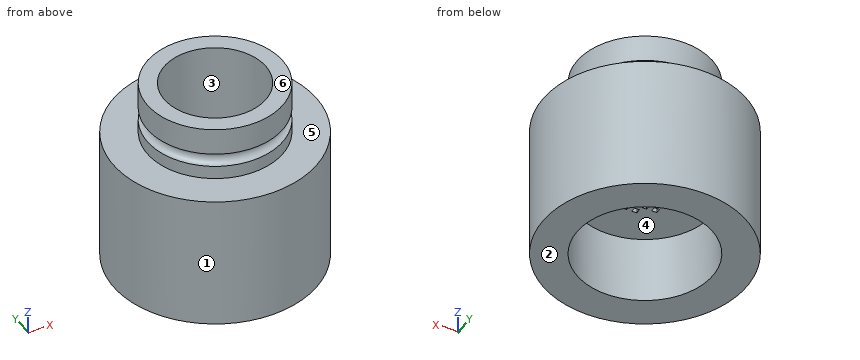
from build123d import *

# Parameters (mm, degrees)
SKETCH1_R                  = 15
BOSS_EXTRUDE1_DEPTH        = 10
SKETCH2_R                  = 10
CUT_EXTRUDE1_DEPTH         = 20
SKETCH3_R                  = 15
BOSS_EXTRUDE2_DEPTH        = 10
SKETCH5_R                  = 10
CUT_EXTRUDE3_DEPTH         = 8
SKETCH8_W                  = 0.75
SKETCH8_H                  = 0.75
CUT_EXTRUDE5_DEPTH         = 2
FILL_START                 = -1.125
FILL_PATTERN2_OUTLINE_W    = 0.75
FILL_PATTERN2_OUTLINE_H    = 2
FILL_PATTERN2_DEPTH        = 0.75
FILL_START_2               = 0.375
FILL_PATTERN2_2_OUTLINE_W  = 0.75
FILL_PATTERN2_2_OUTLINE_H  = 2
FILL_PATTERN2_2_DEPTH      = 0.75
FILL_START_3               = -3.375
FILL_PATTERN2_3_OUTLINE_W  = 0.75
FILL_PATTERN2_3_OUTLINE_H  = 2
FILL_PATTERN2_3_DEPTH      = 0.75
FILL_START_4               = -1.875
FILL_PATTERN2_4_OUTLINE_W  = 0.75
FILL_PATTERN2_4_OUTLINE_H  = 2
FILL_PATTERN2_4_DEPTH      = 0.75
FILL_START_5               = 1.125
FILL_PATTERN2_5_OUTLINE_W  = 0.75
FILL_PATTERN2_5_OUTLINE_H  = 2
FILL_PATTERN2_5_DEPTH      = 0.75
FILL_START_6               = 2.625
FILL_PATTERN2_6_OUTLINE_W  = 0.75
FILL_PATTERN2_6_OUTLINE_H  = 2
FILL_PATTERN2_6_DEPTH      = 0.75
FILL_START_7               = -4.125
FILL_PATTERN2_7_OUTLINE_W  = 0.75
FILL_PATTERN2_7_OUTLINE_H  = 2
FILL_PATTERN2_7_DEPTH      = 0.75
FILL_START_8               = -2.625
FILL_PATTERN2_8_OUTLINE_W  = 0.75
FILL_PATTERN2_8_OUTLINE_H  = 2
FILL_PATTERN2_8_DEPTH      = 0.75
FILL_START_9               = -0.375
FILL_PATTERN2_9_OUTLINE_W  = 0.75
FILL_PATTERN2_9_OUTLINE_H  = 2
FILL_PATTERN2_9_DEPTH      = 0.75
FILL_START_10              = 1.875
FILL_PATTERN2_10_OUTLINE_W = 0.75
FILL_PATTERN2_10_OUTLINE_H = 2
FILL_PATTERN2_10_DEPTH     = 0.75
FILL_START_11              = 3.375
FILL_PATTERN2_11_OUTLINE_W = 0.75
FILL_PATTERN2_11_OUTLINE_H = 2
FILL_PATTERN2_11_DEPTH     = 0.75
SKETCH15_W                 = 16
SKETCH15_H                 = 2.5
SKETCH16_R                 = 1


# Read off the part's stored shape, not the designer's step: Fill Pattern2
with BuildPart() as part:
    # Sketch1 → Boss-Extrude1 (new body)
    with BuildSketch(Plane.XY):
        Circle(SKETCH1_R)
    extrude(amount=BOSS_EXTRUDE1_DEPTH)

    # Sketch2 → Cut-Extrude1 (cut)
    with BuildSketch(Plane.XY.offset(10)):
        Circle(SKETCH2_R)
    extrude(amount=-CUT_EXTRUDE1_DEPTH, mode=Mode.SUBTRACT)

    # Sketch3 → Boss-Extrude2 (add)
    with BuildSketch(Plane.XY.offset(10)):
        Circle(SKETCH3_R)
    extrude(amount=BOSS_EXTRUDE2_DEPTH)

    # Sketch5 → Cut-Extrude3 (cut)
    with BuildSketch(Plane.XY.offset(20)):
        Circle(SKETCH5_R)
    extrude(amount=-CUT_EXTRUDE3_DEPTH, mode=Mode.SUBTRACT)

    # Sketch8 → Cut-Extrude5 (cut)
    with BuildSketch(Plane(origin=(0, 0, 10), x_dir=(-1, 0, 0), z_dir=(0, 0, -1))):
        Rectangle(SKETCH8_W, SKETCH8_H)
    extrude(amount=-CUT_EXTRUDE5_DEPTH, mode=Mode.SUBTRACT)

    # Fill Pattern2 outline → Fill Pattern2 (cut)
    with BuildSketch(Plane.YZ.offset(FILL_START)):
        with Locations((-1.299038106, 11)):
            Rectangle(FILL_PATTERN2_OUTLINE_W, FILL_PATTERN2_OUTLINE_H)
        with Locations((1.299038106, 11)):
            Rectangle(FILL_PATTERN2_OUTLINE_W, FILL_PATTERN2_OUTLINE_H)
        with Locations((-3.897114317, 11)):
            Rectangle(FILL_PATTERN2_OUTLINE_W, FILL_PATTERN2_OUTLINE_H)
        with Locations((3.897114317, 11)):
            Rectangle(FILL_PATTERN2_OUTLINE_W, FILL_PATTERN2_OUTLINE_H)
    extrude(amount=FILL_PATTERN2_DEPTH, mode=Mode.SUBTRACT)

    # Fill Pattern2 2 outline → Fill Pattern2 2 (cut)
    with BuildSketch(Plane.YZ.offset(FILL_START_2)):
        with Locations((-1.299038106, 11)):
            Rectangle(FILL_PATTERN2_2_OUTLINE_W, FILL_PATTERN2_2_OUTLINE_H)
        with Locations((1.299038106, 11)):
            Rectangle(FILL_PATTERN2_2_OUTLINE_W, FILL_PATTERN2_2_OUTLINE_H)
        with Locations((-3.897114317, 11)):
            Rectangle(FILL_PATTERN2_2_OUTLINE_W, FILL_PATTERN2_2_OUTLINE_H)
        with Locations((3.897114317, 11)):
            Rectangle(FILL_PATTERN2_2_OUTLINE_W, FILL_PATTERN2_2_OUTLINE_H)
    extrude(amount=FILL_PATTERN2_2_DEPTH, mode=Mode.SUBTRACT)

    # Fill Pattern2 3 outline → Fill Pattern2 3 (cut)
    with BuildSketch(Plane.YZ.offset(FILL_START_3)):
        with Locations((0, 11)):
            Rectangle(FILL_PATTERN2_3_OUTLINE_W, FILL_PATTERN2_3_OUTLINE_H)
        with Locations((-2.598076211, 11)):
            Rectangle(FILL_PATTERN2_3_OUTLINE_W, FILL_PATTERN2_3_OUTLINE_H)
        with Locations((2.598076211, 11)):
            Rectangle(FILL_PATTERN2_3_OUTLINE_W, FILL_PATTERN2_3_OUTLINE_H)
    extrude(amount=FILL_PATTERN2_3_DEPTH, mode=Mode.SUBTRACT)

    # Fill Pattern2 4 outline → Fill Pattern2 4 (cut)
    with BuildSketch(Plane.YZ.offset(FILL_START_4)):
        with Locations((0, 11)):
            Rectangle(FILL_PATTERN2_4_OUTLINE_W, FILL_PATTERN2_4_OUTLINE_H)
        with Locations((-2.598076211, 11)):
            Rectangle(FILL_PATTERN2_4_OUTLINE_W, FILL_PATTERN2_4_OUTLINE_H)
        with Locations((2.598076211, 11)):
            Rectangle(FILL_PATTERN2_4_OUTLINE_W, FILL_PATTERN2_4_OUTLINE_H)
    extrude(amount=FILL_PATTERN2_4_DEPTH, mode=Mode.SUBTRACT)

    # Fill Pattern2 5 outline → Fill Pattern2 5 (cut)
    with BuildSketch(Plane.YZ.offset(FILL_START_5)):
        with Locations((0, 11)):
            Rectangle(FILL_PATTERN2_5_OUTLINE_W, FILL_PATTERN2_5_OUTLINE_H)
        with Locations((-2.598076211, 11)):
            Rectangle(FILL_PATTERN2_5_OUTLINE_W, FILL_PATTERN2_5_OUTLINE_H)
        with Locations((2.598076211, 11)):
            Rectangle(FILL_PATTERN2_5_OUTLINE_W, FILL_PATTERN2_5_OUTLINE_H)
    extrude(amount=FILL_PATTERN2_5_DEPTH, mode=Mode.SUBTRACT)

    # Fill Pattern2 6 outline → Fill Pattern2 6 (cut)
    with BuildSketch(Plane.YZ.offset(FILL_START_6)):
        with Locations((0, 11)):
            Rectangle(FILL_PATTERN2_6_OUTLINE_W, FILL_PATTERN2_6_OUTLINE_H)
        with Locations((-2.598076211, 11)):
            Rectangle(FILL_PATTERN2_6_OUTLINE_W, FILL_PATTERN2_6_OUTLINE_H)
        with Locations((2.598076211, 11)):
            Rectangle(FILL_PATTERN2_6_OUTLINE_W, FILL_PATTERN2_6_OUTLINE_H)
    extrude(amount=FILL_PATTERN2_6_DEPTH, mode=Mode.SUBTRACT)

    # Fill Pattern2 7 outline → Fill Pattern2 7 (cut)
    with BuildSketch(Plane.YZ.offset(FILL_START_7)):
        with Locations((-1.299038106, 11)):
            Rectangle(FILL_PATTERN2_7_OUTLINE_W, FILL_PATTERN2_7_OUTLINE_H)
        with Locations((1.299038106, 11)):
            Rectangle(FILL_PATTERN2_7_OUTLINE_W, FILL_PATTERN2_7_OUTLINE_H)
    extrude(amount=FILL_PATTERN2_7_DEPTH, mode=Mode.SUBTRACT)

    # Fill Pattern2 8 outline → Fill Pattern2 8 (cut)
    with BuildSketch(Plane.YZ.offset(FILL_START_8)):
        with Locations((-1.299038106, 11)):
            Rectangle(FILL_PATTERN2_8_OUTLINE_W, FILL_PATTERN2_8_OUTLINE_H)
        with Locations((1.299038106, 11)):
            Rectangle(FILL_PATTERN2_8_OUTLINE_W, FILL_PATTERN2_8_OUTLINE_H)
    extrude(amount=FILL_PATTERN2_8_DEPTH, mode=Mode.SUBTRACT)

    # Fill Pattern2 9 outline → Fill Pattern2 9 (cut)
    with BuildSketch(Plane.YZ.offset(FILL_START_9)):
        with Locations((-2.598076211, 11)):
            Rectangle(FILL_PATTERN2_9_OUTLINE_W, FILL_PATTERN2_9_OUTLINE_H)
        with Locations((2.598076211, 11)):
            Rectangle(FILL_PATTERN2_9_OUTLINE_W, FILL_PATTERN2_9_OUTLINE_H)
    extrude(amount=FILL_PATTERN2_9_DEPTH, mode=Mode.SUBTRACT)

    # Fill Pattern2 10 outline → Fill Pattern2 10 (cut)
    with BuildSketch(Plane.YZ.offset(FILL_START_10)):
        with Locations((-1.299038106, 11)):
            Rectangle(FILL_PATTERN2_10_OUTLINE_W, FILL_PATTERN2_10_OUTLINE_H)
        with Locations((1.299038106, 11)):
            Rectangle(FILL_PATTERN2_10_OUTLINE_W, FILL_PATTERN2_10_OUTLINE_H)
    extrude(amount=FILL_PATTERN2_10_DEPTH, mode=Mode.SUBTRACT)

    # Fill Pattern2 11 outline → Fill Pattern2 11 (cut)
    with BuildSketch(Plane.YZ.offset(FILL_START_11)):
        with Locations((-1.299038106, 11)):
            Rectangle(FILL_PATTERN2_11_OUTLINE_W, FILL_PATTERN2_11_OUTLINE_H)
        with Locations((1.299038106, 11)):
            Rectangle(FILL_PATTERN2_11_OUTLINE_W, FILL_PATTERN2_11_OUTLINE_H)
    extrude(amount=FILL_PATTERN2_11_DEPTH, mode=Mode.SUBTRACT)

    # Sketch15 → Revolve2 (revolve)
    with BuildSketch(Plane(origin=(0, 0, 0), x_dir=(0, 0, -1), z_dir=(1, 0, 0)), mode=Mode.PRIVATE) as revolve2_sk:
        with Locations((-20, -8.75)):
            Rectangle(SKETCH15_W, SKETCH15_H)
    revolve(revolve2_sk.sketch.rotate(Axis((0, 0, 20), (0, 0, -1)), 270), axis=Axis((0, 0, 20), (0, 0, -1)))

    # Sketch16 → Cut-Revolve2 (revolve, cut)
    with BuildSketch(Plane(origin=(0, 0, 0), x_dir=(0, 0, -1), z_dir=(1, 0, 0)), mode=Mode.PRIVATE) as cut_revolve2_sk:
        with Locations((-23, 10)):
            Circle(SKETCH16_R)
    revolve(cut_revolve2_sk.sketch.rotate(Axis((0, 0, 20), (0, 0, -1)), 90), axis=Axis((0, 0, 20), (0, 0, -1)), mode=Mode.SUBTRACT)


solid = part.part
Source: CAD feature listing. Evaluate the final solid. Frame: model axes, mm. Face numbers are marked on the shaded views. A direction names the side the tool comes from. Give positions to 0.01 mm unless a question says otherwise; leave off trailing zeros. Write each loop counter-clockwise with the first axis right and the second up, starting at its lowest first coordinate (ties: lowest second). Pieces come first, ordered by that corner, then holes. Notation, with made-up numbers: M 24,58.5 L 37,58.5 A30 cw 37,95.5 Z; hole C 64,-33.5 d2. An arc over 180 degrees is marked long. Return JSON: item names as keys, results as strings. Group by question number.
1) Cut plane A-A, the plane z = 13.5. Output: boundary loops of the cut face in (x, y), then the cut area to 3 significant figures.
2) First-contact query: pin 1 Ø6 at (x, z) = (-12, 20) entering from -Y; pin 2 Ø0.6 at (x, z) = (-3, 10.5) entering from -Y (3 decimals); pin 3 Ø6 at (x, z) = (3.5, 12.5) entering from +Y. Flat tips, straight axial feed; report the tip coordinate or a pass-through.
3) Ray query, L1, parallel to X at y = -0.25, z = 8; L2, parallel to X at y = 0.25, z = 16.75. Return the intervals inside material, ascending.
4) Cut plane B-B, the plane z = 5.5. Output: boundary loops of the cut face in (x, y), then the cut area to 3 significant figures.
5) Set-up query: the marked faces 4, 5 and 6. Return all of +Z, -Z, +X, -X, +Y, -Y with unobstructed straight access to the full face (end or side cutting, diameter ignored); none if empty.
6) Cut plane C-C, the plane y = -12.5. Output: boundary loops of the cut face in (x, z), then the cut area to 3 significant figures.
7) Draft query along Y for the marked faces 1, 2 and 3. Return one class per face: released by +Y, released by -Y, zero draft, split by the parting line, or undercut.
Data:
{
 "1": {"outline": "C 0,0 d30; hole C 0,0 d15", "area": "530 mm²"},
 "2": {"pin 1": "stops at y = -12", "pin 2": "stops at y = -14.755", "pin 3": "stops at y = 14.99"},
 "3": {"L1": "x = -15 to -10, 10 to 15", "L2": "x = -15 to -7.5, 7.5 to 15"},
 "4": {"outline": "C 0,0 d30; hole C 0,0 d20", "area": "393 mm²"},
 "5": {"face 4": "-Z", "face 5": "+Z", "face 6": "+Z, +X, -X, +Y, -Y"},
 "6": {"outline": "M -8.29,0 L 8.29,0 L 8.29,20 L -8.29,20 Z", "area": "332 mm²"},
 "7": {"face 1": "split by the parting line", "face 2": "zero draft", "face 3": "undercut"}
}
